Read the model definition and answer for the solid it produces. Units are mm, in the model's axes. A direction names the side the tool comes from. Coordinates: 2 decimals unless noted, no trailing zeros. Write each loop counter-clockwise with the first axis right and the second up, starting at its lowest first coordinate (ties: lowest second). Pieces come first, ordered by that corner, then holes.
(1) Section C-C on x = -16.6 is taken. Write down the section's boundary in (y, z), then the cut area to 3 significant figures.
(2) The mould has two halves that part along Z. Classify faces 6 (the flat face through (-33, 6, 0)), 7 (the cylindrical face through (40.4, 2.03, -22.43)), 8 (the flat face through (0, 9, 18)), 9 (the flat face through (15, 26, 0)): +Z half, -Z half, draft (parallel to the pull), parting line (faces both ways), or undercut.
(3) Which of the six approach directions +Z, -Z, +X, -X, +Y, -Y give full straight-line access (tool end or side, diameter ignored) to faces 1 (the flat face through (33.5, 9, 0)), 2 (the flat face through (-33.5, 9, 0)), 3 (the cylindrical face through (10.463, 20.423, -1.03)), 4 (the cylindrical face through (32.9, 8.56, -17.43)), 5 (the flat face through (33, 6, 0))?
(4) Given pin 1 (6.5 mm diameter, centred on x = -6, y = 9, fed in from +Z); pin 2 (6 mm diameter, centred on x = -6.5, z = 3.5, fed in from +Y); pin 3 (4 mm diameter, centred on x = 8, y = 5, fed in from -Z); pin 4 (10 mm diameter, centred on x = -16, y = 22, fed in from +Z), each flat-ended and moving along its own axis, determine where each tip first touches the part or whether it passes through.
(5) Section D-D on x = 15.1 is taken. Write down the section's boundary in (y, z).
(6) Section A-A on x = 37.5 is taken. Write down the section's boundary in (y, z), then the cut area to 3 significant figures.
(7) Section B-B on y = 5 is taken. Write down the section's boundary in (x, z), then the cut area to 3 significant figures.
(8) Find the intervals of material crossed by probe 1 along Z at (x, y) = (-37.5, 2.7); probe 2 along X at (y, z) = (3.25, 8.75); probe 3 along Z at (x, y) = (26.5, 2.5), in increasing order.
from build123d import *

# Parameters (mm, degrees)
ESQUISSE1_W             = 82
ESQUISSE1_H             = 46
ESQUISSE1_R             = 3
BOSS_EXTRU_1_DEPTH      = 15
ESQUISSE2_W             = 66
ESQUISSE2_H             = 31
ENL_V_MAT_EXTRU_1_DEPTH = 13
ENL_V_START             = 15
ESQUISSE3_R             = 8.75
ENL_V_MAT_EXTRU_2_DEPTH = 65.345719166
ESQUISSE4_W             = 67
ESQUISSE4_H             = 36
ENL_V_MAT_EXTRU_3_DEPTH = 11
BOSS_EXTRU_3_START      = 15
ESQUISSE5_R             = 4.75
BOSS_EXTRU_3_DEPTH      = 11
ENL_V_START_2           = 4
ESQUISSE1_4_W           = 60
ESQUISSE1_4_H           = 1
ENL_V_MAT_EXTRU_4_DEPTH = 1
CONG_1_R                = 2
CONG_2_R                = 2
CONG_4_R                = 2


with BuildPart() as part:
    # Esquisse1 → Boss.-Extru.1 (new body)
    with BuildSketch(Plane(origin=(0, 0, 0), x_dir=(1, 0, 0), z_dir=(0, 1, 0))):
        Rectangle(ESQUISSE1_W, ESQUISSE1_H)
        with Locations(Location((-37.5, 8.75, 0), (0, 0, 270))):
            Circle(ESQUISSE1_R, mode=Mode.SUBTRACT)
        with Locations(Location((37.5, 8.75, 0), (0, 0, 270))):
            Circle(ESQUISSE1_R, mode=Mode.SUBTRACT)
        with Locations(Location((37.5, -8.75, 0), (0, 0, 270))):
            Circle(ESQUISSE1_R, mode=Mode.SUBTRACT)
        with Locations(Location((-37.5, -8.75, 0), (0, 0, 270))):
            Circle(ESQUISSE1_R, mode=Mode.SUBTRACT)
    extrude(amount=BOSS_EXTRU_1_DEPTH)

    # Esquisse2 → Enlèv. mat.-Extru.1 (cut)
    with BuildSketch(Plane(origin=(0, 0, 0), x_dir=(1, 0, 0), z_dir=(0, 1, 0))):
        Rectangle(ESQUISSE2_W, ESQUISSE2_H)
    extrude(amount=ENL_V_MAT_EXTRU_1_DEPTH, mode=Mode.SUBTRACT)

    # Esquisse3 → Enlèv. mat.-Extru.2 (cut, through all)
    with BuildSketch(Plane(origin=(0, 0, 0), x_dir=(1, 0, 0), z_dir=(0, 1, 0)).offset(ENL_V_START)):
        with Locations(Location((-16.6, 0, 0), (0, 0, 270))):
            Circle(ESQUISSE3_R)
    extrude(amount=-ENL_V_MAT_EXTRU_2_DEPTH, mode=Mode.SUBTRACT)

    # Esquisse4 → Enlèv. mat.-Extru.3 (cut)
    with BuildSketch(Plane(origin=(0, 0, 0), x_dir=(1, 0, 0), z_dir=(0, 1, 0)).offset(ENL_V_START)):
        Polygon((-33.5, -23), (-41, -23), (-41, 23), (-33.5, 23), (33.5, 23), (41, 23), (41, -23), (33.5, -23), align=None)
        Rectangle(ESQUISSE4_W, ESQUISSE4_H, mode=Mode.SUBTRACT)
    extrude(amount=-ENL_V_MAT_EXTRU_3_DEPTH, mode=Mode.SUBTRACT)

    # Esquisse5 → Boss.-Extru.3 (add)
    with BuildSketch(Plane(origin=(0, 0, 0), x_dir=(1, 0, 0), z_dir=(0, 1, 0)).offset(BOSS_EXTRU_3_START)):
        with Locations(Location((15.1, 0, 0), (0, 0, 270))):
            Circle(ESQUISSE5_R)
    extrude(amount=BOSS_EXTRU_3_DEPTH)

    # Esquisse1<4> → Enlèv. mat.-Extru.4 (cut)
    with BuildSketch(Plane(origin=(0, 0, 0), x_dir=(1, 0, 0), z_dir=(0, 1, 0)).offset(ENL_V_START_2)):
        with Locations((0, -21)):
            Rectangle(ESQUISSE1_4_W, ESQUISSE1_4_H)
        with Locations((0, 21)):
            Rectangle(ESQUISSE1_4_W, ESQUISSE1_4_H)
    extrude(amount=-ENL_V_MAT_EXTRU_4_DEPTH, mode=Mode.SUBTRACT)

    # Congé1
    cong_1_edges = [part.edges().sort_by_distance(p)[0] for p in [
        (0, 15, 18),
        (-33.5, 15, 0),
        (0, 15, -18),
        (33.5, 15, 0),
    ]]
    fillet(cong_1_edges, radius=CONG_1_R)

    # Congé2
    # the kernel refuses this fillet: 2 mm, written as the material it takes off along each edge
    with BuildSketch(Plane(origin=(-31.5, 13, -16), x_dir=(0, 0, -1), z_dir=(-1, 0, 0))) as cong_2_piece_1_section:
        Polygon((0, 0), (CONG_2_R, 0), (CONG_2_R, -CONG_2_R), (0, -CONG_2_R), align=None)
    cong_2_piece_1 = extrude(amount=CONG_2_R, mode=Mode.PRIVATE)
    cong_2_piece_1 = cong_2_piece_1 - Plane(origin=(-31.5, 13, -16), x_dir=(0, -0.7071067811865475, 0.7071067811865475), z_dir=(-1, 0, 0)) * Sphere(CONG_2_R, mode=Mode.PRIVATE)
    add(cong_2_piece_1, mode=Mode.SUBTRACT)
    with BuildSketch(Plane(origin=(-31.5, 13, 16), x_dir=(-1, 0, 0), z_dir=(0, 0, 1))) as cong_2_piece_2_section:
        Polygon((0, 0), (CONG_2_R, 0), (CONG_2_R, -CONG_2_R), (0, -CONG_2_R), align=None)
    cong_2_piece_2 = extrude(amount=CONG_2_R, mode=Mode.PRIVATE)
    cong_2_piece_2 = cong_2_piece_2 - Plane(origin=(-31.5, 13, 16), x_dir=(0.7071067811865475, -0.7071067811865475, 0), z_dir=(0, 0, 1)) * Sphere(CONG_2_R, mode=Mode.PRIVATE)
    add(cong_2_piece_2, mode=Mode.SUBTRACT)
    with BuildSketch(Plane(origin=(31.5, 13, -16), x_dir=(0, 0, -1), z_dir=(1, 0, 0))) as cong_2_piece_3_section:
        Polygon((0, 0), (CONG_2_R, 0), (CONG_2_R, CONG_2_R), (0, CONG_2_R), align=None)
    cong_2_piece_3 = extrude(amount=CONG_2_R, mode=Mode.PRIVATE)
    cong_2_piece_3 = cong_2_piece_3 - Plane(origin=(31.5, 13, -16), x_dir=(0, -0.7071067811865475, 0.7071067811865475), z_dir=(1, 0, 0)) * Sphere(CONG_2_R, mode=Mode.PRIVATE)
    add(cong_2_piece_3, mode=Mode.SUBTRACT)
    with BuildSketch(Plane(origin=(31.5, 13, 16), x_dir=(1, 0, 0), z_dir=(0, 0, 1))) as cong_2_piece_4_section:
        Polygon((0, 0), (CONG_2_R, 0), (CONG_2_R, CONG_2_R), (0, CONG_2_R), align=None)
    cong_2_piece_4 = extrude(amount=CONG_2_R, mode=Mode.PRIVATE)
    cong_2_piece_4 = cong_2_piece_4 - Plane(origin=(31.5, 13, 16), x_dir=(-0.7071067811865475, -0.7071067811865475, 0), z_dir=(0, 0, 1)) * Sphere(CONG_2_R, mode=Mode.PRIVATE)
    add(cong_2_piece_4, mode=Mode.SUBTRACT)
    with BuildSketch(Plane(origin=(-33.5, 13, 18), x_dir=(1, 0, 0), z_dir=(0, -1, 0)), Plane(origin=(-33.5, 13, -18), x_dir=(0, 0, 1), z_dir=(0, -1, 0))) as cong_2_piece_5:
        with BuildLine():
            CenterArc((CONG_2_R, -CONG_2_R), CONG_2_R, 90, 90)
            Line((0, -CONG_2_R), (0, 0))
            Line((0, 0), (CONG_2_R, 0))
        make_face()
    extrude(amount=9, mode=Mode.SUBTRACT)
    with BuildSketch(Plane(origin=(33.5, 13, -18), x_dir=(0, 0, 1), z_dir=(0, -1, 0)), Plane(origin=(33.5, 13, 18), x_dir=(-1, 0, 0), z_dir=(0, -1, 0))) as cong_2_piece_6:
        with BuildLine():
            CenterArc((CONG_2_R, CONG_2_R), CONG_2_R, 180, 90)
            Line((0, CONG_2_R), (0, 0))
            Line((0, 0), (CONG_2_R, 0))
        make_face()
    extrude(amount=9, mode=Mode.SUBTRACT)

    # Congé4
    cong_4_edges = [part.edges().sort_by_distance(p)[0] for p in [
        (41, 2, 23),
        (-41, 2, 23),
        (-41, 2, -23),
        (41, 2, -23),
    ]]
    fillet(cong_4_edges, radius=CONG_4_R)


solid = part.part
Response:
1. outline: (0, -23) - (4, -23) - (4, -21.5) - (3, -21.5) - (3, -20.5) - (4, -20.5) - (4, -18) - (13, -18) arc R2 ccw to (15, -16) - (15, -8.75) - (13, -8.75) - (13, -15.5) - (0, -15.5) - close; (0, 15.5) - (13, 15.5) - (13, 8.75) - (15, 8.75) - (15, 16) arc R2 ccw to (13, 18) - (4, 18) - (4, 20.5) - (3, 20.5) - (3, 21.5) - (4, 21.5) - (4, 23) - (0, 23) - close
1. area: 138 mm2
2. face 6: undercut
2. face 7: -Z half
2. face 8: +Z half
2. face 9: draft
3. face 1: +Z, -Z, +X, +Y
3. face 2: +Z, -Z, -X, +Y
3. face 3: +Y
3. face 4: -Z, +X, +Y
3. face 5: -Y
4. pin 1: stops at z = 18
4. pin 2: stops at y = 15
4. pin 3: stops at z = -23
4. pin 4: passes through
5. outline: (0, -23) - (4, -23) - (4, -21.5) - (3, -21.5) - (3, -20.5) - (4, -20.5) - (4, -18) - (13, -18) arc R2 ccw to (15, -16) - (15, -4.75) - (26, -4.75) - (26, 4.75) - (15, 4.75) - (15, 16) arc R2 ccw to (13, 18) - (4, 18) - (4, 20.5) - (3, 20.5) - (3, 21.5) - (4, 21.5) - (4, 23) - (0, 23) - (0, 15.5) - (13, 15.5) - (13, -15.5) - (0, -15.5) - close
6. outline: (0, -23) - (4, -23) - (4, -11.75) - (0, -11.75) - close; (0, -5.75) - (4, -5.75) - (4, 5.75) - (0, 5.75) - close; (0, 11.75) - (4, 11.75) - (4, 23) - (0, 23) - close
6. area: 136 mm2
7. outline: (-33.5, -16) arc R2 ccw to (-31.5, -18) - (31.5, -18) arc R2 ccw to (33.5, -16) - (33.5, 16) arc R2 ccw to (31.5, 18) - (-31.5, 18) arc R2 ccw to (-33.5, 16) - close; hole (-33, -15.5) - (33, -15.5) - (33, 15.5) - (-33, 15.5) - close
7. area: 363 mm2
8. probe 1: z = -23 to -11.75, -5.75 to 5.75, 11.75 to 23
8. probe 2: x = -41 to -40.5, -34.5 to -33, 33 to 34.5, 40.5 to 41
8. probe 3: z = -23 to -15.5, 15.5 to 23
